Build history of the part. All positions in model axes, mm. Give positions to 0.01 mm unless a question says otherwise; leave off trailing zeros. Write each loop counter-clockwise with the first axis right and the second up, starting at its lowest first coordinate (ties: lowest second). Pieces come first, ordered by that corner, then holes.
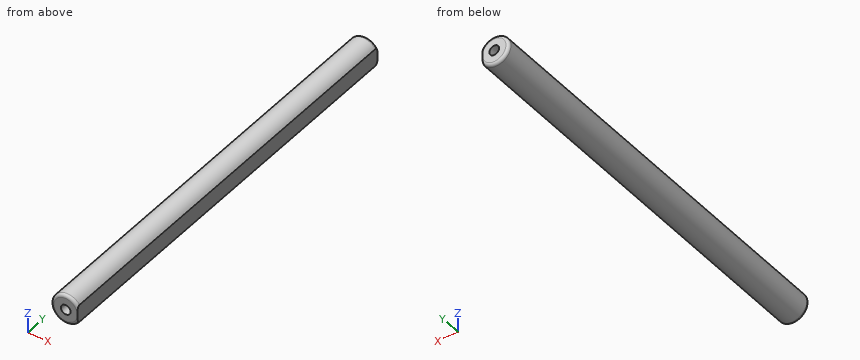
from build123d import *

# Parameters (mm, degrees)
SKETCH1_R            = 2.5
BOSS_EXTRUDE1_DEPTH  = 35.15
SKETCH2_R            = 0.825
CUT_EXTRUDE1_DEPTH   = 5
CUT_EXTRUDE2_DEPTH   = 36.327361917
FILLET1_R            = 0.5
FILLET1_OF_MIRROR1_R = 0.5


with BuildPart() as part:
    # Sketch1 → Boss-Extrude1 (new body)
    with BuildSketch(Plane(origin=(0, 0, 0), x_dir=(1, 0, 0), z_dir=(0, 1, 0))):
        with Locations(Location((0, 0, 0), (0, 0, 270))):
            Circle(SKETCH1_R)
    boss_extrude1 = extrude(amount=BOSS_EXTRUDE1_DEPTH)

    # Sketch2 → Cut-Extrude1 (cut)
    with BuildSketch(Plane(origin=(0, 35.15, 0), x_dir=(1, 0, 0), z_dir=(0, 1, 0))):
        with Locations(Location((0, 0, 0), (0, 0, 270))):
            Circle(SKETCH2_R)
    cut_extrude1 = extrude(amount=-CUT_EXTRUDE1_DEPTH, mode=Mode.SUBTRACT)

    # Sketch3 → Cut-Extrude2 (cut, through all)
    with BuildSketch(Plane(origin=(0, 35.15, 0), x_dir=(1, 0, 0), z_dir=(0, 1, 0))):
        with BuildLine():
            Line((2, 1.5), (2, -1.5))
            ThreePointArc((2, -1.5), (2.5, 0), (2, 1.5))
        make_face()
    cut_extrude2 = extrude(amount=-CUT_EXTRUDE2_DEPTH, mode=Mode.SUBTRACT)

    # Fillet1
    fillet1_edges = [part.edges().sort_by_distance(p)[0] for p in [
        (-2.5, 35.15, 0),
    ]]
    fillet(fillet1_edges, radius=FILLET1_R - 0.0001)  # a hair under: the kernel refuses the full size

    # Mirror1: Boss-Extrude1, Cut-Extrude1, Cut-Extrude2 across plane
    add(boss_extrude1.mirror(Plane.ZX))
    add(cut_extrude1.mirror(Plane.ZX), mode=Mode.SUBTRACT)
    add(cut_extrude2.mirror(Plane.ZX), mode=Mode.SUBTRACT)

    # Fillet1 of Mirror1
    fillet1_of_mirror1_edges = [part.edges().sort_by_distance(p)[0] for p in [
        (-2.5, -35.15, 0),
    ]]
    fillet(fillet1_of_mirror1_edges, radius=FILLET1_OF_MIRROR1_R - 0.0001)  # a hair under: the kernel refuses the full size


solid = part.part
1. Saw through at A-A on x = 0. Give the cut face in (y, z) (3 decimals).
2. Drill centre lines: line 1 along X through (y, z) = (-34, 0) (3 decimals); line 2 along Y through (x, z) = (-0.35, 2); line 3 along Y through (x, z) = (0.3, -0.6). Where is each one in solid material? Low to high.
3. Drop flat-ended pins along their axis: pin 1 (1 mm diameter, centred on x = 1, y = -23, fed in from -Z); pin 2 (0.8 mm diameter, centred on x = 0, z = 0, fed in from +Y); pin 3 (1.3 mm diameter, centred on x = 0, z = 0, fed in from -Y). Give the stop position or say it passes through.
4. Saw through at B-B on y = -13. Give the cut face in (x, z), plus the area to 3 significant figures.
Outcome:
1. outline: (-35.15, -2) arc R0.5 ccw to (-34.65, -2.5) - (34.65, -2.5) arc R0.5 ccw to (35.15, -2) - (35.15, -0.825) - (30.15, -0.825) - (30.15, 0.825) - (35.15, 0.825) - (35.15, 2) arc R0.5 ccw to (34.65, 2.5) - (-34.65, 2.5) arc R0.5 ccw to (-35.15, 2) - (-35.15, 0.825) - (-30.15, 0.825) - (-30.15, -0.825) - (-35.15, -0.825) - close
2. line 1: x = -2.5 to -0.825, 0.825 to 2
2. line 2: y = -35.15 to 35.15
2. line 3: y = -30.15 to 30.15
3. pin 1: stops at z = -2.45
3. pin 2: stops at y = 30.15
3. pin 3: stops at y = -30.15
4. outline: (2, -1.5) - (2, 1.5) arc R2.5 ccw (long way) to start
4. area: 18.6 mm2
